Here's how the part is built. I have some questions about the finished solid (model axes, mm). A direction names the side the tool comes from. Round coordinates to 2 decimals unless told otherwise and drop trailing zeros. Order: outer loops, then holes, each group sorted by start corner. A loop starts at its lowest first (then second) coordinate and runs counter-clockwise, first axis right, second up. Notation, with made-up numbers: (-28, 81.5) -> (9, 81.5) arc R12 ccw to (9, 89.5) -> close; hole circle Ø3 at (-7.75, 3.5). An arc over 180 degrees is marked (long way). Answer in a Markdown table with one row per item.
Autodesk Inventor part; units mm, degrees
ref_plane "Płaszczyzna konstrukcyjna1" through (25, 3, -48.75) normal (1, 0, 0) x (0, 0, 1)
ref_plane "YZ Plane" through (0, 0, 0) normal (1, 0, 0) x (0, 1, 0)
ref_plane "XZ Plane" through (0, 0, 0) normal (0, 1, 0) x (-1, 0, 0)
sketch "Szkic1" plane through (0, 0, 0) normal (0, 1, 0) x (-1, 0, 0)
  line L0 (0, 0) -> (-25, 0)
  line L1 (-25, 0) -> (-25, -110)
  line L2 (-25, -110) -> (0, -110)
  line L3 (0, -110) -> (0, 0)
  line L4 (-4, -2) -> (-25, -2)
  line L5 (-25, -2) -> (-25, -90)
  line L6 (-25, -90) -> (-4, -90)
  line L7 (-4, -90) -> (-4, -2)
  line L8 (-25, -90) -> (-4, -2)
  line L9 (-22, -90) -> (-4, -14.5714)
  line L10 (-4, -14.5714) -> (-4, -2)
  line L11 (-25, -90) -> (-22, -90)
  dimension "d0" = 25
  dimension "d1" = 110
  dimension "d2" = 4
  dimension "d3" = 20
  dimension "d4" = 2
  dimension "d7" = 3
extrude "Wyciągnięcie proste2" add sketch "Szkic1" along normal blind 5 contours L3 L2 L1 L6 L7 L4 L0 | L8 L7 L9 L6
sketch "Szkic2" plane through (25, 0, 0) normal (1, 0, 0) x (0, 0, -1)
  line L0 (0, 0) -> (-33, 0)
  line L1 (-33, 0) -> (-33, 7)
  line L2 (-33, 7) -> (0, 7)
  line L3 (0, 7) -> (0, 0)
  line L4 (-33, 0) -> (-30, 7)
  dimension "d10" = 33
  dimension "d11" = 7
  dimension "d12" = 30
extrude "Wyciągnięcie proste3" add sketch "Szkic2" against normal blind 50 contours L0 L4 L2 L3
sketch "Szkic3" plane through (25, 7, 30) normal (0, 1, 0) x (1, 0, 0)
  line L0 (0, 0) -> (-50, 0)
  line L1 (0, 0) -> (-48.5, 0)
  line L2 (-48.5, 0) -> (-48.5, 28.5)
  line L3 (-48.5, 28.5) -> (0, 28.5)
  line L4 (-50, 0) -> (-50, 30)
  line L5 (-48.5, 28.5) -> (-41.5, 28.5)
  line L6 (-41.5, 28.5) -> (-41.5, 16.5)
  line L7 (-41.5, 16.5) -> (-48.5, 16.5)
  line L8 (-48.5, 16.5) -> (-48.5, 28.5)
  circle A0 centre (-41.5, 22.5) radius 6
  line L9 (-35.5, 22.5) -> (-41.5, 22.5)
  line L10 (-41.5, 22.5) -> (-41.5, 28.5)
  line L11 (-41.5, 28.5) -> (-35.5, 28.5)
  line L12 (-35.5, 28.5) -> (-35.5, 22.5)
  line L13 (0, 30) -> (-50, 30)
  line L14 (0, 30) -> (0, 0)
  line L15 (-19, 28.5) -> (-7, 28.5) construction
  line L16 (-22.5355, 28.5) -> (-19, 28.5)
  line L17 (-7, 28.5) -> (-5, 28.5)
  line L18 (-7, 0) -> (-5, 0)
  point P0 (-25, 30)
  dimension "d16" = 1.5
  dimension "d19" = 13
  dimension "d20" = 12
  dimension "d66" = 1.5
extrude "Wyciągnięcie proste4" cut sketch "Szkic3" against normal up to next contours L0 L2 L7 A0 L12 L3 L14
sketch "Szkic5" plane through (0, 5, 0) normal (0, 1, 0) x (1, 0, 0)
  line L0 (25, 90) -> (25, 110)
  line L1 (0, 110) -> (0, 0)
  line L2 (25, 110) -> (0, 110)
  line L3 (0, 110) -> (0, 85)
  line L4 (0, 85) -> (25, 85)
  line L5 (25, 85) -> (25, 110)
  circle A0 centre (15, 100) radius 3
  dimension "d30" = 25
  dimension "d31" = 6
  dimension "d32" = 10
  dimension "d33" = 10
extrude "Wyciągnięcie proste6" cut sketch "Szkic5" against normal blind 2
chamfer "Faza2" distance 2 distance2 1 1 edges at (12, 3, -100) measured on face at (17.3983, 3.6667, -98.1978)
chamfer "Faza3" distance 2 angle 45 1 edges at (12.5, 5, 0)
sketch "Szkic6" plane through (15, 5, -100) normal (0, 1, 0) x (1, 0, 0)
  point P0 (-15, -100)
  point P1 (0, 0)
hole "Otwór1" at (15, 5, -100) direction (0, -1, 0) diameter 3 end through all
sketch "Szkic7" plane through (-25, 7, 30) normal (0, 1, 0) x (1, 0, 0)
  line L0 (14.5, 28.5) -> (14.5, 22.5) construction
  line L1 (14.5, 28.5) -> (14.5, 20) construction
  line L2 (14.5, 20) -> (1.5, 20) construction
  line L3 (1.5, 16.5) -> (1.5, 0) construction
  line L4 (1.5, 20) -> (1.5, 16.5) construction
  line L5 (1.5, 20) -> (10, 20) construction
  point P0 (25, 30)
  point P1 (14.5, 22.5)
  point P2 (12.5, 27.5)
  dimension "d49" = 8.5
  dimension "d50" = 8.5
hole "Otwór2" at (-15, 7, 10) direction (0, -1, 0) diameter 3 end through all
ref_plane "Płaszczyzna konstrukcyjna1" through (25, 3, -48.75) normal (1, 0, 0) x (0, 0, 1)
mirror "Odbij1" about plane through (25, 3, -48.75) normal (1, 0, 0)
fillet "Fillet1" radius 2 4 edges at (4, 5, -49.7857) (0, 5, -43.4998) (46, 5, -49.7857) (50, 5, -43.4998)
properties part number "lf20cm"
1. We'd pull the mould along X, two halves only. Please class faces 6 (the face through (13.7, 5, -101.3)), 7 (the face through (-12.304, 3.549, 11.789)), 8 (the face through (50, 1, -54)): released by +X, released by -X, zero draft, split by the parting line, or undercut.
Numbers:
| item | result |
|---|---|
| face 6 | zero draft |
| face 7 | undercut |
| face 8 | released by +X |
2. Suppose I cut it at C-C on z = -100. State how many separate pieces and enclosed holes the cut face has, then the cut area to 3 significant figures.
Numbers:
| item | result |
|---|---|
| separate pieces | 3 |
| enclosed holes | 0 |
| area | 148 mm2 |
3. Suppose I cut it at B-B on z = 3. Write out the boundary of the cut face in (x, y), then the cut area to 3 significant figures.
Numbers:
| item | result |
|---|---|
| outline | (-25, 0) -> (-10.5, 0) -> (-10.5, 7) -> (-25, 7) -> close; (60.5, 0) -> (75, 0) -> (75, 7) -> (60.5, 7) -> close |
| area | 203 mm2 |
4. Suppose I cut it at A-A on x = 69. Write out the boundary of the cut face in (y, z).
Numbers:
| item | result |
|---|---|
| outline | (0, 0) -> (7, 0) -> (7, 13.5) -> (0, 13.5) -> close; (0, 30) -> (7, 30) -> (0, 33) -> close |
5. Please list where these lines run through material, in increasing order: line 1 along X through (y, z) = (2.35, -100); line 2 along X through (y, z) = (3.25, 10); line 3 along Z through (x, y) = (65, 4.25).
Numbers:
| item | result |
|---|---|
| line 1 | x = 0 to 13.5, 16.5 to 33.5, 36.5 to 50 |
| line 2 | x = -25 to -16.5, -13.5 to -11.05, 61.05 to 63.5, 66.5 to 75 |
| line 3 | z = 0 to 8.5, 11.5 to 13.31, 30 to 31.18 |
6. For faces 1 (the face through (33.7, 5, -101.3)), 2 (the face through (-23.5, 4, 22)), 3 (the face through (22, 7, 1)), 4 (the face through (59, 4, 0)), 5 (the face through (-25, 4, 17)), which set-ups out of +Z, -Z, +X, -X, +Y, -Y let a thin tool reach every point of the face, with its end or its side?
Numbers:
| item | result |
|---|---|
| face 1 | -Z, +X, -X, +Y |
| face 2 | +Y, -Y |
| face 3 | +Z, -Z, +X, -X, +Y |
| face 4 | -Z, +Y, -Y |
| face 5 | +Z, -Z, -X, +Y, -Y |
7. For pin 1 Ø2 at (x, y) = (32.5, 4.5) entering from -Z; pin 2 Ø3 at (y, z) = (2.5, -18) entering from -X; pin 3 Ø2.5 at (x, z) = (35, -100) entering from -Y; pin 4 Ø3.5 at (y, z) = (1, -53) entering from +X, each with a flat end and sliding along its axis, tell me the tip position at first contact or that it passes through.
Numbers:
| item | result |
|---|---|
| pin 1 | stops at z = -103.13 |
| pin 2 | stops at x = 0 |
| pin 3 | passes through |
| pin 4 | stops at x = 50 |
